The model under review builds one solid part; all positions refer to its coordinate system, in mm. Give positions to 0.01 mm unless a question says otherwise; leave off trailing zeros. Loops run counter-clockwise (first coordinate to the right, second up) from the corner with the lowest first, then second, coordinate; pieces in that order, holes last. Notation, with made-up numbers: M 89,8 L 99,8 A23 cw 99,45 Z; hole C 57,-25 d3. An arc over 180 degrees is marked long. Return JSON: item names as keys, results as strings.
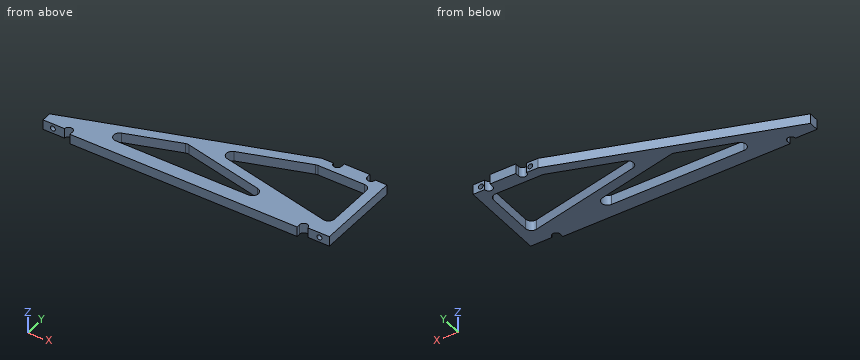
Autodesk Inventor part; units mm, degrees
ref_plane "YZ Plane" through (0, 0, 0) normal (1, 0, 0) x (0, 1, 0)
ref_plane "XZ Plane" through (0, 0, 0) normal (0, 1, 0) x (-1, 0, 0)
ref_plane "XY Plane" through (0, 0, 0) normal (0, 0, 1) x (1, 0, 0)
sketch "スケッチ1" plane through (0, 0, 0) normal (0, 0, 1) x (1, 0, 0)
  line L0 (-72.5, -21.65) -> (72.5, -21.65) construction
  line L1 (72.5, -21.65) -> (72.5, 21.65) construction
  line L2 (72.5, 21.65) -> (-72.5, 21.65) construction
  line L3 (-72.5, 21.65) -> (-72.5, -21.65) construction
  line L4 (-72.5, -21.65) -> (72.5, 21.65) construction
  line L5 (72.5, -21.65) -> (-72.5, 21.65) construction
  line L6 (-67.5, 21.65) -> (-67.5, -21.65) construction
  line L7 (0, 0) -> (0, 21.65) construction
  line L8 (0, 0) -> (-72.5, 0) construction
  line L9 (67.5, 21.65) -> (67.5, -21.65) construction
  line L10 (-72.5, -21.65) -> (-61.6, -21.65)
  line L11 (49.5, 21.65) -> (49.5, 23.65)
  line L12 (49.5, 23.65) -> (62.5, 23.65)
  line L13 (62.5, 23.65) -> (62.5, 21.65)
  line L14 (66.6, 21.65) -> (72.5, 21.65)
  line L15 (72.5, 21.65) -> (72.5, -21.65)
  line L16 (72.5, -21.65) -> (61.6, -21.65)
  line L17 (-57.5, -21.65) -> (-57.5, -23.65)
  line L18 (-57.5, -23.65) -> (57.5, -23.65)
  line L19 (57.5, -23.65) -> (57.5, -21.65)
  arc A0 (45.4, 21.65) -> (49.5, 21.65) centre (47.45, 21.65) ccw
  arc A1 (62.5, 21.65) -> (66.6, 21.65) centre (64.55, 21.65) ccw
  arc A2 (-57.5, -21.65) -> (-61.6, -21.65) centre (-59.55, -21.65) ccw
  arc A3 (61.6, -21.65) -> (57.5, -21.65) centre (59.55, -21.65) ccw
  line L20 (-72.5, -21.65) -> (-72.5, -16.65)
  line L21 (-72.5, -16.65) -> (39.5, 21.65)
  line L22 (45.4, 21.65) -> (39.5, 21.65)
  line L23 (66.95, 24.476) -> (70.05, 24.476) construction
  line L24 (70.05, 24.476) -> (70.05, 13.3235) construction
  line L25 (70.05, 13.3235) -> (66.95, 13.3235) construction
  line L26 (66.95, 13.3235) -> (66.95, 24.476) construction
  line L27 (68.5, 24.476) -> (68.5, 13.3235) construction
  line L28 (41.95, 24.476) -> (45.05, 24.476) construction
  line L29 (45.05, 24.476) -> (45.05, 13.9945) construction
  line L30 (45.05, 13.9945) -> (41.95, 13.9945) construction
  line L31 (41.95, 13.9945) -> (41.95, 24.476) construction
  line L32 (43.5, 24.476) -> (43.5, 13.9945) construction
  dimension "d16" = 5
  dimension "d20" = 43.3
  dimension "d40" = 135
  dimension "d41" = 10
  dimension "d42" = 2.05
  dimension "d43" = 2
  dimension "d44" = 5
  dimension "d45" = 10
  dimension "d46" = 10
  dimension "d48" = 3.1
  dimension "d50" = 4
  dimension "d51" = 25
  dimension "d52" = 3.1
  dimension "d62" = 6
  dimension "d63" = 6
extrude "押し出し1" add sketch "スケッチ1" along normal blind 2.5
mirror "ミラー1" about plane through (8.3734, -6.8299, 0) normal (0, 0, -1) of "押し出し1"
sketch "スケッチ2" plane through (-72.5, -21.65, 2.5) normal (0, -1, 0) x (1, 0, 0)
  line L0 (0, -5) -> (0, 0)
  line L1 (15, -5) -> (130, -5) construction
  line L2 (72.5, -5) -> (72.5, 0) construction
  line L3 (15, 0) -> (130, 0) construction
  point P0 (72.5, -2.5)
  point P1 (5, -2.5)
  point P2 (140, -2.5)
  point P3 (0, -2.5)
  dimension "d26" = 5
hole "穴1" at (-67.5, -21.65, 0) at (67.5, -21.65, 0) direction (0, 1, 0) diameter 2.459 depth 2
sketch "スケッチ4" plane through (66.6, 21.65, 2.5) normal (0, 1, 0) x (1, 0, 0)
  line L0 (5.9, 5) -> (5.9, 0)
  point P0 (-66.6, 2.5)
  point P1 (1.9, 2.5)
  point P2 (-23.1, 2.5)
  point P3 (5.9, 2.5)
  dimension "d53" = 4
  dimension "d54" = 25
hole "穴2" at (68.5, 21.65, 0) at (43.5, 21.65, 0) direction (0, -1, 0) diameter 2.459 depth 2.5
sketch "スケッチ6" plane through (0, 0, 2.5) normal (0, 0, 1) x (1, 0, 0)
  line L0 (61.6, -21.65) -> (72.5, -21.65)
  line L1 (72.5, -21.65) -> (72.5, 21.65)
  line L2 (72.5, 21.65) -> (66.6, 21.65)
  line L3 (39.5, 21.65) -> (-72.5, -16.65)
  line L4 (67.5, 16.65) -> (67.5, -16.65) construction
  line L5 (67.5, -16.65) -> (-57.0473, -16.65) construction
  line L6 (-57.0473, -16.65) -> (40.3313, 16.65) construction
  line L7 (40.3313, 16.65) -> (67.5, 16.65) construction
  line L8 (67.5, -16.65) -> (-8.358, 0) construction
  line L9 (67.5, -14.0905) -> (67.5, 16.65)
  line L10 (67.5, 16.65) -> (40.3313, 16.65)
  line L11 (40.3313, 16.65) -> (-3.7993, 1.5589)
  line L12 (-3.7993, 1.5589) -> (67.5, -14.0905)
  line L13 (55.8388, -16.65) -> (-57.0473, -16.65)
  line L14 (-57.0473, -16.65) -> (-12.9167, -1.5589)
  line L15 (-12.9167, -1.5589) -> (55.8388, -16.65)
  point P0 (0, 0)
  dimension "d72" = 5
  dimension "d73" = 5
  dimension "d74" = 5
  dimension "d75" = 5
  dimension "d76" = 5
extrude "押し出し4" cut sketch "スケッチ6" against normal blind 10
fillet "フィレット3" radius 3 7 edges at (-3.7993, 1.5589, 0) (40.3313, 16.65, 0) (67.5, -14.0905, 0) (55.8388, -16.65, 0) (-12.9167, -1.5589, 0) (-57.0473, -16.65, 0) (67.5, 16.65, 0)
equation "\"d16\" = d4"
equation "\"d40\" = d6"
equation "\"d41\" = d3"
equation "\"d46\" = d45"
equation "\"d63\" = d62"
equation "\"d73\" = d72"
equation "\"d74\" = d73"
equation "\"d75\" = d74"
equation "\"d76\" = d74"
properties part number "前腕_サブフレーム_1_1" material "アセタール樹脂、黒"
1) Consider section D-D on z = 0. Count the separate pieces of the cut face and the enclosed holes in it, then the cut area to 3 significant figures.
From the geometry:
{"separate pieces": "1", "enclosed holes": "2", "area": "2,330 mm²"}
2) Consider section B-B on y = -5.5. Write out the cut boundary in (x, z), then the cut area to 3 significant figures.
From the geometry:
{"outline": "M -39.89,-2.5 L -24.44,-2.5 L -24.44,2.5 L -39.89,2.5 Z; M 5.04,-2.5 L 28.36,-2.5 L 28.36,2.5 L 5.04,2.5 Z; M 67.5,-2.5 L 72.5,-2.5 L 72.5,2.5 L 67.5,2.5 Z", "area": "219 mm²"}
3) Insertion check: pin 1 (2 mm diameter, centred on x = 68, z = -0.5, fed in from +Y); pin 2 (0.6 mm diameter, centred on y = 22.5, z = 1, fed in from +X); pin 3 (1.5 mm diameter, centred on x = -11, z = -0.5, fed in from +Y). Each pin has a flat end and moves straight along its axis. Give the tip position at first contact, or say it passes through.
From the geometry:
{"pin 1": "y = 21.65", "pin 2": "x = 62.5", "pin 3": "y = 4.64"}
4) Consider section C-C on x = 26.5. Write out the cut boundary in (y, z).
From the geometry:
{"outline": "M -23.65,-2.5 L -16.65,-2.5 L -16.65,2.5 L -23.65,2.5 Z; M -10.21,-2.5 L -5.09,-2.5 L -5.09,2.5 L -10.21,2.5 Z; M 11.92,-2.5 L 17.2,-2.5 L 17.2,2.5 L 11.92,2.5 Z"}
5) Consider section A-A on x = 47.45. Write out the cut boundary in (y, z), then the cut area to 3 significant figures.
From the geometry:
{"outline": "M -23.65,-2.5 L -9.69,-2.5 L -9.69,2.5 L -23.65,2.5 Z; M 16.65,-2.5 L 19.6,-2.5 L 19.6,2.5 L 16.65,2.5 Z", "area": "84.6 mm²"}
6) Wall thickness on L1, parallel to Y at x = 26, z = 1; L2, parallel to Y at x = 11.5, z = -1.4 (3 decimals); L3, parallel to Z at x = -67.5, y = -20.7: over which ranges is each line inside the solid? List them lowest first. Write a range as from..to.
From the geometry:
{"L1": "-23.65..-16.65, -10.1..-4.98, 11.75..17.03", "L2": "-23.65..-16.65, -6.918..-1.799, 6.791..12.075", "L3": "-2.5..-1.23, 1.23..2.5"}
